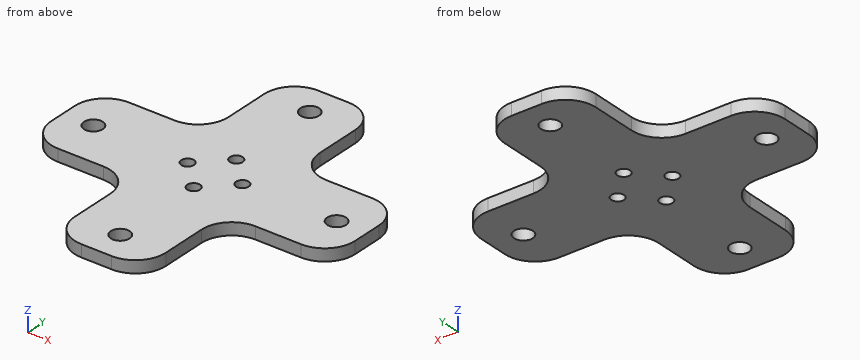
from build123d import *

# Parameters (mm, degrees)
F0_W            = 15
F0_H            = 17.5
F0_H_2          = 15
F0_W_2          = 17.5
F1_DEPTH        = 2
F2_R            = 1.05
F2_R_2          = 1.55
F3_DEPTH        = 25
F3_COPIES_COUNT = 4
F4_R            = 5


# Not quite as in the source:
# - a pattern or mirror of a feature is missing from the dataset's text; its kind, count and spacing are read off the source's solid


with BuildPart() as f1:
    # F0 (on Top) → F1 (new body)
    with BuildSketch(Plane.XY):
        with Locations((0, 16.25)):
            Rectangle(F0_W, F0_H)
        Rectangle(F0_W, F0_H_2)
        with Locations((-16.25, 0)):
            Rectangle(F0_W_2, F0_H_2)
        with Locations((16.25, 0)):
            Rectangle(F0_W_2, F0_H_2)
        with Locations((0, -16.25)):
            Rectangle(F0_W, F0_H)
    extrude(amount=F1_DEPTH)

    # F2 (on face) → F3 (cut)
    with BuildSketch(Plane.XY.offset(2)):
        with Locations((-4.5, 0)):
            Circle(F2_R)
        with Locations((-20, 0)):
            Circle(F2_R_2)
    f3 = extrude(amount=-F3_DEPTH, mode=Mode.SUBTRACT)

    # F3_copies: F3 ×4 about axis
    f3_copies_axis = Axis((0, 0, 0), (0, 0, 1))
    for i in range(1, F3_COPIES_COUNT):
        add(f3.rotate(f3_copies_axis, i * 360 / F3_COPIES_COUNT), mode=Mode.SUBTRACT)

    # F4
    f4_edges = [f1.edges().sort_by_distance(p)[0] for p in [
        (7.5, -25, 1),
        (-7.5, -25, 1),
        (-7.5, -7.5, 1),
        (-25, -7.5, 1),
        (-25, 7.5, 1),
        (-7.5, 7.5, 1),
        (-7.5, 25, 1),
        (7.5, 25, 1),
        (25, 7.5, 1),
        (7.5, 7.5, 1),
        (25, -7.5, 1),
        (7.5, -7.5, 1),
    ]]
    fillet(f4_edges, radius=F4_R)


solid = f1.part
The model under review builds one solid part; all positions refer to its coordinate system, in mm. Coordinates: 2 decimals unless noted, no trailing zeros. Write each loop counter-clockwise with the first axis right and the second up, starting at its lowest first coordinate (ties: lowest second). Pieces come first, ordered by that corner, then holes. Notation, with made-up numbers: (67.5, 53) -> (77.5, 53) arc R6 ccw to (77.5, 64) -> close; hole circle Ø8 at (-3, -23.75). An arc over 180 degrees is marked (long way). Answer in a Markdown table with one row per item.
1. Clearance check with flat-ended pins moving along their axes: pin 1 Ø1 at (x, z) = (-16.5, 0.5) entering from -Y; pin 2 Ø0.6 at (y, z) = (-18, 1.5) entering from -X; pin 3 Ø1 at (y, z) = (17, 1.5) entering from +X. State where each tip first meets the part, or that it passes through.
Answers below:
| item | result |
|---|---|
| pin 1 | stops at y = -7.5 |
| pin 2 | stops at x = -7.5 |
| pin 3 | stops at x = 7.5 |
2. We need section B-B, the plane y = -4.5. State the section outline as (x, z) points, and give its area (3 significant figures).
Answers below:
| item | result |
|---|---|
| outline | (-24.58, 0) -> (-1.05, 0) -> (-1.05, 2) -> (-24.58, 2) -> close; (1.05, 0) -> (24.58, 0) -> (24.58, 2) -> (1.05, 2) -> close |
| area | 94.1 mm^2 |
3. We need section C-C, the plane z = 0.5. Give the number of separate pieces and of enclosed holes in the cut face, and give its area (3 significant figures).
Answers below:
| item | result |
|---|---|
| separate pieces | 1 |
| enclosed holes | 8 |
| area | 1,210 mm^2 |
4. We need section D-D, the plane x = 15.5. State the section outline as (y, z) points.
Answers below:
| item | result |
|---|---|
| outline | (-7.5, 0) -> (7.5, 0) -> (7.5, 2) -> (-7.5, 2) -> close |
5. We need section A-A, the plane x = 0. State the section outline as (y, z) points, and give its area (3 significant figures).
Answers below:
| item | result |
|---|---|
| outline | (-25, 0) -> (-21.55, 0) -> (-21.55, 2) -> (-25, 2) -> close; (-18.45, 0) -> (-5.55, 0) -> (-5.55, 2) -> (-18.45, 2) -> close; (-3.45, 0) -> (3.45, 0) -> (3.45, 2) -> (-3.45, 2) -> close; (5.55, 0) -> (18.45, 0) -> (18.45, 2) -> (5.55, 2) -> close; (21.55, 0) -> (25, 0) -> (25, 2) -> (21.55, 2) -> close |
| area | 79.2 mm^2 |
6. Wall thickness on probe 1 along X at (y, z) = (20, 0.6); probe 2 along Y at (x, z) = (13.5, 1.95): over which ranges is each line inside the solid? List them lowest first. Write a range as [from, to].
Answers below:
| item | result |
|---|---|
| probe 1 | x = [-7.5, -1.55], [1.55, 7.5] |
| probe 2 | y = [-7.5, 7.5] |
